Model file for the job. Use its own axes, mm. Face numbers are marked on the shaded views. A direction names the side the tool comes from. Round coordinates to 2 decimals unless told otherwise and drop trailing zeros. Loops run counter-clockwise (first coordinate to the right, second up) from the corner with the lowest first, then second, coordinate; pieces in that order, holes last. Notation, with made-up numbers: M -15.75,74.5 L -3.75,74.5 A35 cw -3.75,106.5 Z; hole C 5.25,12.5 d6. An arc over 180 degrees is marked long. Use a Markdown table: item, result. Add a question column.
Q1. Cut at C-C (y = 23). Give the cut face in (x, z) (3 decimals).
Q2. Tool access for the marked faces 1, 2, 3, 4 and 5: list every direction of +Z, -Z, +X, -X, +Y, -Y with a clear straight run to the whole face (end or side of a thin tool).
Q3. Cut at B-B (z = -3.5). Give the cut face in (x, y), plus the area to 3 significant figures.
Q4. Probe line 1 (Z direction, x = -0.75, y = 16.75); line 2 (Y direction, x = 0.75, z = -3); line 3 (Y direction, x = -3, z = 0.5). List the from-to ranges inside material, lowest first. Write a range as from..to.
Q5. Cut at A-A (x = 4.5). Give the cut face in (y, z), plus the area to 3 significant figures.
Q6. Cut at D-D (y = 11). Give the cut face in (x, z) (3 decimals), plus the area to 3 significant figures.
Q7. Mould opens along Y. For the marked faces 6, 7 and 8 say: +Y half, -Y half, draft (parallel to the pull), parting line (faces both ways), or undercut.
Q8. Pin check, flat tips, straight feed: pin 1 (1.7 mm diameter, centred on y = 2.5, z = 2, fed in from +X); pin 2 (0.6 mm diameter, centred on x = 7, z = -0.5, fed in from +Y); pin 3 (2 mm diameter, centred on x = 5.5, z = 4, fed in from +Y); pin 4 (2 mm diameter, centred on x = 5.5, y = 16, fed in from -Z). Stop position of each tip, or through.
Autodesk Inventor part; units mm, degrees
ref_plane "YZ Plane" through (0, 0, 0) normal (1, 0, 0) x (0, 1, 0)
ref_plane "XZ Plane" through (0, 0, 0) normal (0, 1, 0) x (-1, 0, 0)
ref_plane "XY Plane" through (0, 0, 0) normal (0, 0, 1) x (1, 0, 0)
sketch "Sketch1" plane through (0, 0, 0) normal (0, 1, 0) x (-1, 0, 0)
  line L0 (-6.35, 5.5563) -> (-6.35, -5.5563)
  line L1 (-6.35, -5.5563) -> (6.35, -5.5563)
  line L2 (6.35, -5.5563) -> (6.35, 5.5563)
  line L3 (6.35, 5.5563) -> (-6.35, 5.5563)
  line L4 (-6.35, 5.5563) -> (6.35, -5.5563) construction
  line L5 (-6.35, -5.5563) -> (6.35, 5.5563) construction
  point P0 (0, 0)
  dimension "d0" = 11.1125
  dimension "d1" = 12.7
extrude "Extrusion1" add sketch "Sketch1" along normal blind 6.35
sketch "Sketch3" plane through (0, 6.35, 0) normal (0, 1, 0) x (1, 0, 0)
  circle A0 centre (0, 0) radius 3.175
  dimension "d8" = 6.35
extrude "Extrusion3" add sketch "Sketch3" along normal blind 6.35
thread "Thread1"
sketch "Sketch4" plane through (6.35, 0, 5.5563) normal (1, 0, 0) x (0, 0, -1)
  line L0 (4.7625, 4.7625) -> (6.35, 4.7625)
  line L1 (6.35, 4.7625) -> (6.35, 7.9375)
  line L2 (6.35, 7.9375) -> (4.7625, 7.9375)
  line L3 (4.7625, 7.9375) -> (4.7625, 4.7625)
  line L4 (0, 6.35) -> (11.1125, 6.35)
  line L5 (4.7625, 4.7625) -> (6.35, 7.9375) construction
  line L6 (6.35, 4.7625) -> (4.7625, 7.9375) construction
  point P0 (5.5563, 0)
  point P1 (5.5563, 6.35)
  dimension "d13" = 1.5875
  dimension "d14" = 3.175
extrude "Extrusion4" add sketch "Sketch4" along normal blind 0.7937
sketch "Sketch5" plane through (0, 12.7, 0) normal (0, 1, 0) x (1, 0, 0)
  circle A0 centre (0, 0) radius 2.54
  dimension "d17" = 5.08
extrude "Extrusion5" add sketch "Sketch5" along normal blind 0.7937
sketch "Sketch6" plane through (0, 13.4938, 0) normal (0, 1, 0) x (1, 0, 0)
  circle A0 centre (0, 0) radius 3.175
extrude "Extrusion6" add sketch "Sketch6" along normal blind 12.7
sketch "Sketch7" plane through (0, 26.1938, 0) normal (0, 1, 0) x (1, 0, 0)
  line L0 (-3.175, -0.3969) -> (3.175, -0.3969)
  line L1 (3.175, -0.3969) -> (3.175, 0.3969)
  line L2 (3.175, 0.3969) -> (-3.175, 0.3969)
  line L3 (-3.175, 0.3969) -> (-3.175, -0.3969)
  line L4 (-3.175, -0.3969) -> (3.175, 0.3969) construction
  line L5 (3.175, -0.3969) -> (-3.175, 0.3969) construction
  point P0 (0, 0)
  dimension "d22" = 0.7937
extrude "Extrusion7" cut sketch "Sketch7" against normal blind 11.1125
sketch "Sketch8" plane through (3.1501, 26.1938, 0.3969) normal (0, 0, -1) x (-1, 0, 0)
  point P0 (3.1501, -26.1938)
sketch "Sketch9" plane through (0, 15.0813, 0) normal (0, 1, 0) x (1, 0, 0)
  circle A0 centre (0, 0) radius 3.175
  circle A1 centre (0, 0) radius 2.3813
  dimension "d25" = 4.7625
extrude "Extrusion8" cut sketch "Sketch9" along normal blind 1.5875
chamfer "Chamfer1" distance 0.7937 angle 45 3 edges at (0, 16.6687, 3.175) (0, 16.6687, -3.175) (-3.175, 15.0813, 0)
chamfer "Chamfer2" distance 0.7937 angle 45 2 edges at (0, 26.1938, 3.175) (0, 26.1938, -3.175)
fillet "Fillet1" radius 0.7937 11 edges at (0, 6.35, -5.5563) (-6.35, 6.35, 0) (-6.35, 3.175, -5.5563) (0, 0, -5.5563) (6.35, 0, 0) (6.35, 3.175, 5.5563) (0, 6.35, 5.5563) (6.35, 3.175, -5.5563) (0, 0, 5.5563) (-6.35, 3.175, 5.5563) (-6.35, 0, 0)
properties part number "stepped-encoder"
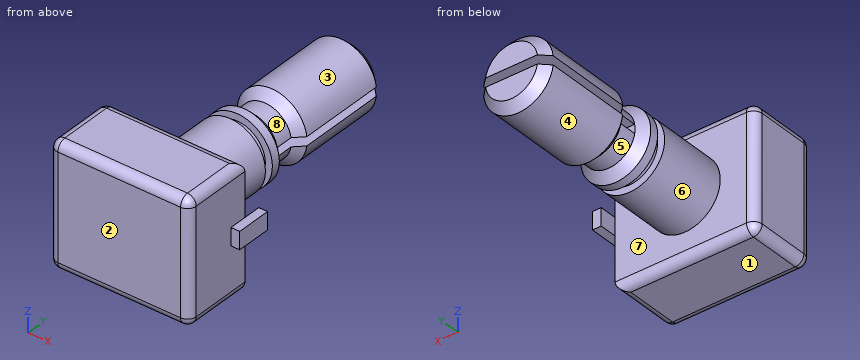
Checked values:
| question | item | result |
|---|---|---|
| 1 | outline | M -3.15,-0.397 A3.175 ccw 3.15,-0.397 Z; M -3.15,0.397 L 3.15,0.397 A3.175 ccw Z |
| 2 | face 1 | -Z, +X, -X, +Y, -Y |
| 2 | face 2 | +Z, -Z, +X, -X, -Y |
| 2 | face 3 | +Z, +Y |
| 2 | face 4 | -Z, +Y |
| 2 | face 5 | -Z |
| 3 | outline | M -6.35,0.79 A0.79 ccw -5.56,0 L 5.56,0 A0.79 ccw 6.35,0.79 L 6.35,6.35 L -5.56,6.35 A0.79 ccw -6.35,5.56 Z |
| 3 | area | 80.2 mm^2 |
| 4 | line 1 | z = -2.35..-0.4, 0.4..2.35 |
| 4 | line 2 | y = 0..12.7, 13.49..14.37, 17.38..25.48 |
| 4 | line 3 | y = 0..12.7, 13.49..14.42, 17.33..25.53 |
| 5 | outline | M 0,-4.76 A0.79 ccw 0.79,-5.56 L 5.56,-5.56 A0.79 ccw 6.35,-4.76 L 6.35,4.76 A0.79 ccw 5.56,5.56 L 0.79,5.56 A0.79 ccw 0,4.76 Z |
| 5 | area | 70.0 mm^2 |
| 6 | outline | C 0,0 d6.35 |
| 6 | area | 31.7 mm^2 |
| 7 | face 6 | draft |
| 7 | face 7 | +Y half |
| 7 | face 8 | undercut |
| 8 | pin 1 | stops at x = 6.35 |
| 8 | pin 2 | stops at y = 7.94 |
| 8 | pin 3 | stops at y = 6.35 |
| 8 | pin 4 | passes through |
